The model under review builds one solid part; all positions refer to its coordinate system, in mm. Face numbers are marked on the shaded views. A direction names the side the tool comes from. Coordinates: 2 decimals unless noted, no trailing zeros. Loops run counter-clockwise (first coordinate to the right, second up) from the corner with the lowest first, then second, coordinate; pieces in that order, holes last. Notation, with made-up numbers: M 82.5,-5 L 100.5,-5 A21 cw 100.5,7 Z; hole C 62.25,76.25 d11. An arc over 180 degrees is marked long. Return JSON: item names as keys, results as strings.
```python
from build123d import *

# Parameters (mm, degrees)
SKETCH1_R           = 5
BOSS_EXTRUDE1_DEPTH = 135
BOSS_EXTRUDE2_START = -100
SKETCH3_R           = 7.5
SKETCH3_R_2         = 5
BOSS_EXTRUDE2_DEPTH = 2
FILLET1_R           = 1


with BuildPart() as part:
    # Sketch1 → Boss-Extrude1 (new body)
    with BuildSketch(Plane(origin=(0, 0, 0), x_dir=(1, 0, 0), z_dir=(0, 1, 0))):
        with Locations(Location((0, 0, 0), (0, 0, 270))):
            Circle(SKETCH1_R)
    extrude(amount=BOSS_EXTRUDE1_DEPTH)

    # Sketch2 → Revolve3 (revolve)
    with BuildSketch(Plane.XY, mode=Mode.PRIVATE) as revolve3_sk:
        Polygon((0, 145), (5, 135), (0, 135), align=None)
    revolve(revolve3_sk.sketch.rotate(Axis((0, 135, 0), (0, -1, 0)), 270), axis=Axis((0, 135, 0), (0, -1, 0)))

    # Sketch3 → Boss-Extrude2 (add)
    with BuildSketch(Plane.XZ.offset(BOSS_EXTRUDE2_START)):
        with Locations(Location((0, 0, 0), (0, 0, 270))):
            Circle(SKETCH3_R)
        with Locations(Location((0, 0, 0), (0, 0, 270))):
            Circle(SKETCH3_R_2, mode=Mode.SUBTRACT)
    extrude(amount=-BOSS_EXTRUDE2_DEPTH)

    # Fillet1
    fillet1_edges = [part.edges().sort_by_distance(p)[0] for p in [
        (0, 100, 7.5),
        (0, 102, 7.5),
    ]]
    fillet(fillet1_edges, radius=FILLET1_R - 0.0001)  # a hair under: the kernel refuses the full size


solid = part.part
```
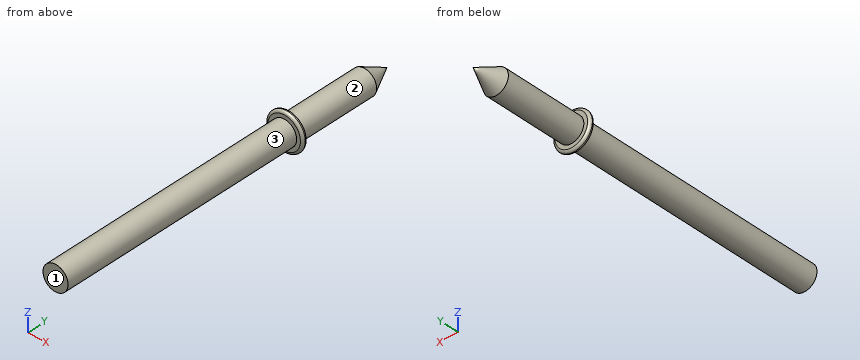
1. Machinability: for the marked faces 1, 2 and 3, which of the approach directions +Z, -Z, +X, -X, +Y, -Y give a long, thin tool a straight path to every point of the face, cutting with its end or side? Answer none if there is none.
Check values:
{"face 1": "+Z, -Z, +X, -X, -Y", "face 2": "+Y", "face 3": "-Y"}
2. Insertion check: pin 1 Ø5 at (x, z) = (-5.5, -5.5) entering from +Y; pin 2 Ø2 at (x, y) = (-5, 59.5) entering from -Z; pin 3 Ø1 at (x, y) = (-1, 27.5) entering from -Z. Each pin has a flat end and moves straight along its axis. Give the tip position at first contact, or say it passes through.
Check values:
{"pin 1": "y = 102", "pin 2": "z = -3", "pin 3": "z = -4.97"}
3. To check wall thickness, follow line 1 (Y direction, x = -5.75, z = 1.75); line 2 (X direction, y = 7.5, z = -1.75); line 3 (X direction, y = 55.5, z = 3.5). State the ranges of each line that lie inside material, in increasing order.
Check values:
{"line 1": "100 to 102", "line 2": "-4.68 to 4.68", "line 3": "-3.57 to 3.57"}
4. Add section A-A on y = 95.5. Give the boundary of the cut face in (x, z), plus the area to 3 significant figures.
Check values:
{"outline": "C 0,0 d10", "area": "78.5 mm²"}
